Geometry check sheet. Reference: the model listing, model coordinates, mm. A direction names the side the tool comes from. Round coordinates to 2 decimals unless told otherwise and drop trailing zeros. Write each loop counter-clockwise with the first axis right and the second up, starting at its lowest first coordinate (ties: lowest second). Pieces come first, ordered by that corner, then holes.
Item 1: Cross-section at D-D (z = 6.5). Enter the section's corners in (x, y) (1 decimal).
Item 2: Access from +Z, -Z, +X, -X, +Y, -Y to the whole of each face (thin tool, end or side, straight path). Record for faces 1 (the face through (0, 8, 10.16)), 2 (the face through (-3.92, 7.79, 10.35)), 3 (the face through (3.87, 7.7, 10.35)), 4 (the face through (0, -4.949, 19)), 5 (the face through (0, 8, 25.4)).
Item 3: Cross-section at A-A (x = -0.5). Enter the section's corners in (y, z), then the cut area to 3 significant figures.
Item 4: Depth check by flat-ended pin: P1, Ø1.5, axis at x = 0.5, y = -22, coming from the -Z side; P2, Ø1, axis at x = -2, z = 34.5, coming from the +Y side; P3, Ø5, axis at x = 4.5, y = -35.5, coming from the +Z side; P4, Ø4.5, axis at x = 0, z = 10.5, coming from the +Y side. Enter the tip coordinate at first touch or a pass-through.
Item 5: Draft check along Y on faces 6 (the face through (4.306, 2.44, 12.522)), 7 (the face through (0, 4.949, 7)), 8 (the face through (4.266, -46.959, 69.761)), 9 (the face through (0.04, -17.59, 44.72)). Enter one of: pulls with the +Y half, pulls with the -Y half, needs draft (parallel to the pull), parting line crosses it, or undercut.
Item 6: Scan lines: probe 1 along Y at (x, z) = (3, 22.5); probe 2 along Z at (x, y) = (4.5, -25); probe 3 along Z at (x, y) = (3.25, 3). Record each from-to range of solid material in increasing order.
from build123d import *

# Parameters (mm, degrees)
BOSS_EXTRUDE1_DEPTH = 25.4
BOSS_EXTRUDE2_DEPTH = 12.7
BOSS_EXTRUDE3_DEPTH = 25.4
CHAMFER1_SIZE       = 7.46
CHAMFER1_SIZE2      = 12.54
CUT_EXTRUDE1_DEPTH  = 10.16
CUT_EXTRUDE3_DEPTH  = 83.695754046
CHAMFER7_SIZE       = 0.381


with BuildPart() as part:
    # Sketch1 → Boss-Extrude1 (new body)
    with BuildSketch(Plane.XY):
        Polygon((5.715, 0), (2.8575, 4.949335183), (-2.8575, 4.949335183), (-5.715, 0), (-2.8575, -4.949335183), (2.8575, -4.949335183), align=None)
    extrude(amount=BOSS_EXTRUDE1_DEPTH)



with BuildPart() as body_2:
    # Sketch2 → Boss-Extrude2 (new body)
    with BuildSketch(Plane.XY.offset(63.5)):
        Polygon((-2.8575, -49.399335183), (2.8575, -49.399335183), (5.715, -44.45), (2.8575, -39.500664817), (-2.8575, -39.500664817), (-5.715, -44.45), align=None)
    extrude(amount=BOSS_EXTRUDE2_DEPTH)


with BuildPart() as part_1:
    add(part.part)

    add(body_2.part)  # loft1 joins it to this body
    # loft from a face of the part (loft1)
    loft([part_1.faces().sort_by_distance((0, 0, 25.4))[0], part_1.faces().sort_by_distance((0, -44.45, 63.5))[0]])

    # Sketch4 → Boss-Extrude3 (add)
    with BuildSketch(Plane(origin=(0, 0, 0), x_dir=(-1, 0, 0), z_dir=(0, 0, -1))):
        Polygon((2.8575, 4.949335183), (6.083733304, 10.537335183), (-6.083733304, 10.537335183), (-2.8575, 4.949335183), align=None)
    extrude(amount=-BOSS_EXTRUDE3_DEPTH)

    # Chamfer1
    chamfer1_edges = [part_1.edges().sort_by_distance(p)[0] for p in [
        (0, -4.949335183, 0),
    ]]
    chamfer1_side = [part_1.faces().sort_by_distance(p)[0] for p in [
        (0, 2.994180076, 0),
    ]]
    chamfer(chamfer1_edges, length=CHAMFER1_SIZE, length2=CHAMFER1_SIZE2, reference=chamfer1_side[0])

    # Sketch8 → Cut-Extrude1 (cut)
    with BuildSketch(Plane(origin=(0, 0, 0), x_dir=(-1, 0, 0), z_dir=(0, 0, -1))):
        Polygon((-6.083733304, 10.537335183), (6.083733304, 10.537335183), (2.8575, 4.949335183), (-2.8575, 4.949335183), align=None)
    extrude(amount=-CUT_EXTRUDE1_DEPTH, mode=Mode.SUBTRACT)

    # Sketch9 → Cut-Extrude3 (cut, through all)
    with BuildSketch(Plane(origin=(0, 0, 10.16), x_dir=(-1, 0, 0), z_dir=(0, 0, -1))):
        Polygon((5.728133304, 10.537335183), (2.5019, 4.949335183), (2.8575, 4.949335183), (6.083733304, 10.537335183), align=None)
        Polygon((-2.5019, 4.949335183), (-5.728133304, 10.537335183), (-6.083733304, 10.537335183), (-2.8575, 4.949335183), align=None)
    extrude(amount=-CUT_EXTRUDE3_DEPTH, mode=Mode.SUBTRACT)

    # Chamfer7
    chamfer7_edges = [part_1.edges().sort_by_distance(p)[0] for p in [
        (4.115016652, 7.743335183, 10.16),
        (-4.115016652, 7.743335183, 10.16),
        (0, 10.537335183, 10.16),
    ]]
    chamfer(chamfer7_edges, length=CHAMFER7_SIZE)


solid = part_1.part
Resolved:
1. outline: (-5.7, 0) - (-4.9, -1.4) - (4.9, -1.4) - (5.7, 0) - (2.9, 4.9) - (-2.9, 4.9) - close
2. face 1: -Z, +X, -X, +Y
2. face 2: -Z, -X
2. face 3: -Z, +X
2. face 4: -Z, +X, -X, -Y
2. face 5: +Z, +X, -X, +Y
3. outline: (-49.4, 63.5) - (-4.95, 25.4) - (-4.95, 12.54) - (2.51, 0) - (4.95, 0) - (4.95, 10.16) - (10.16, 10.16) - (10.54, 10.54) - (10.54, 25.4) - (4.95, 25.4) - (-39.5, 63.5) - (-39.5, 76.2) - (-49.4, 76.2) - close
3. area: 793 mm2
4. P1: stops at z = 39.37
4. P2: stops at y = -5.08
4. P3: stops at z = 61.69
4. P4: stops at y = 10.54
5. face 6: undercut
5. face 7: undercut
5. face 8: pulls with the -Y half
5. face 9: pulls with the +Y half
6. probe 1: y = -4.7 to 4.7, 5.81 to 10.54
6. probe 2: z = 45.02 to 48.63
6. probe 3: z = 0 to 26.49
